Geometry: final body of the model. Coordinates: model frame, mm. A direction names the side the tool comes from. Round coordinates to 2 decimals unless told otherwise and drop trailing zeros. Write each loop counter-clockwise with the first axis right and the second up, starting at its lowest first coordinate (ties: lowest second). Pieces come first, ordered by that corner, then holes. Notation, with made-up numbers: (38.5, 73.5) -> (85.5, 73.5) arc R22 cw to (85.5, 91.5) -> close; hole circle Ø8 at (27, 78). An arc over 180 degrees is marked (long way). One line per item, written item: value. Start each with the question number.
from build123d import *

# Parameters (mm, degrees)
SKETCH1_W           = 50
SKETCH1_H           = 50
BOSS_EXTRUDE1_DEPTH = 2
BOSS_EXTRUDE2_DEPTH = 8
FILLET1_R           = 10
CUT_EXTRUDE1_DEPTH  = 1


with BuildPart() as part:
    # Sketch1 → Boss-Extrude1 (new body)
    with BuildSketch(Plane(origin=(0, 0, 0), x_dir=(1, 0, 0), z_dir=(0, 1, 0))):
        with Locations((-178.886902591, -23.537255169)):
            Rectangle(SKETCH1_W, SKETCH1_H)
    extrude(amount=BOSS_EXTRUDE1_DEPTH)

    # Sketch2 → Boss-Extrude2 (add)
    with BuildSketch(Plane(origin=(0, 2, 0), x_dir=(1, 0, 0), z_dir=(0, 1, 0))):
        with BuildLine():
            Line((-189.683230088, -36.437255169), (-193.090575095, -36.437255169))
            ThreePointArc((-193.090575095, -36.437255169), (-191.386902591, -37.787255169), (-189.683230088, -36.437255169))
        make_face()
        with BuildLine():
            Line((-193.090575095, -35.637255169), (-191.386902591, -35.637255169))
            Line((-191.386902591, -35.637255169), (-189.683230088, -35.637255169))
            ThreePointArc((-189.683230088, -35.637255169), (-191.386902591, -34.287255169), (-193.090575095, -35.637255169))
        make_face()
        with BuildLine():
            Line((-168.090575095, -35.637255169), (-166.386902591, -35.637255169))
            Line((-166.386902591, -35.637255169), (-164.683230088, -35.637255169))
            ThreePointArc((-164.683230088, -35.637255169), (-166.386902591, -34.287255169), (-168.090575095, -35.637255169))
        make_face()
        with BuildLine():
            Line((-164.683230088, -36.437255169), (-168.090575095, -36.437255169))
            ThreePointArc((-168.090575095, -36.437255169), (-166.386902591, -37.787255169), (-164.683230088, -36.437255169))
        make_face()
        with BuildLine():
            Line((-193.346494385, -10.637255169), (-191.386902591, -10.637255169))
            Line((-191.386902591, -10.637255169), (-189.427310797, -10.637255169))
            ThreePointArc((-189.427310797, -10.637255169), (-191.386902591, -9.037255169), (-193.346494385, -10.637255169))
        make_face()
        with BuildLine():
            Line((-189.427310797, -11.437255169), (-193.346494385, -11.437255169))
            ThreePointArc((-193.346494385, -11.437255169), (-191.386902591, -13.037255169), (-189.427310797, -11.437255169))
        make_face()
        with BuildLine():
            Line((-168.346494385, -10.637255169), (-166.386902591, -10.637255169))
            Line((-166.386902591, -10.637255169), (-164.427310797, -10.637255169))
            ThreePointArc((-164.427310797, -10.637255169), (-166.386902591, -9.037255169), (-168.346494385, -10.637255169))
        make_face()
        with BuildLine():
            Line((-164.427310797, -11.437255169), (-168.346494385, -11.437255169))
            ThreePointArc((-168.346494385, -11.437255169), (-166.386902591, -13.037255169), (-164.427310797, -11.437255169))
        make_face()
    extrude(amount=BOSS_EXTRUDE2_DEPTH)

    # Fillet1
    fillet1_edges = [part.edges().sort_by_distance(p)[0] for p in [
        (-203.886902591, 1, -1.462744831),
        (-153.886902591, 1, -1.462744831),
        (-153.886902591, 1, 48.537255169),
        (-203.886902591, 1, 48.537255169),
    ]]
    fillet(fillet1_edges, radius=FILLET1_R)

    # Sketch3 → Cut-Extrude1 (cut)
    with BuildSketch(Plane(origin=(0, 2, 0), x_dir=(1, 0, 0), z_dir=(0, 1, 0))):
        Polygon((-177.886902591, -47.537255169), (-178.886902591, -47.537255169), (-179.886902591, -47.537255169), (-179.886902591, -48.537255169), (-177.886902591, -48.537255169), align=None)
    extrude(amount=-CUT_EXTRUDE1_DEPTH, mode=Mode.SUBTRACT)


solid = part.part
(1) Pin query (flat end, axial travel): pin 1 (3.5 mm diameter, centred on x = -191, y = 5, fed in from +Z); pin 2 (0.8 mm diameter, centred on y = 1.5, z = 48, fed in from -X); pin 3 (4 mm diameter, centred on x = -174.5, y = 4.5, fed in from -Z); pin 4 (1 mm diameter, centred on y = 3.5, z = 34, fed in from +X). Return the tip coordinate at first contact, or that it passes through.
(2) Section query B-B (z = 31.5). Output: boundary loops of the cut face in (x, y), and give its area (3 significant figures).
(3) Section query A-A (y = 8.5). Output: boundary loops of the cut face in (x, z).
(4) Pull-direction query (Z, two-part tool) for faces 1 (the face through (-179, 1, -1.463)), 2 (the face through (-191.354, 5.944, 34.288)), 3 (the face through (-166, 10, 35)), 4 (the face through (-201.035, 1.014, 45.53)); classes: pulls with the +Z half, pulls with the -Z half, needs draft (parallel to the pull), parting line crosses it, or undercut.
(5) Section query C-C (x = -180.5). Output: boundary loops of the cut face in (y, z).
(6) Set-up query: faces 5 (the face through (-191, 6, 13)), 6 (the face through (-179.1, 0.8, 48.537)), 7 (the face through (-191, 6, 36.437)). Return all of +Z, -Z, +X, -X, +Y, -Y with unobstructed straight access to the full face (end or side cutting, diameter ignored); none if empty.
(7) Line query: probe 1 along Z at (x, y) = (-192, 4.75); probe 2 along Y at (x, z) = (-183.5, 16); probe 3 along Z at (x, y) = (-167.5, 6). Output: solid intervals per line, ascending.
Results list:
1. pin 1: stops at z = 37.79
1. pin 2: stops at x = -198.11
1. pin 3: passes through
1. pin 4: stops at x = -165.55
2. outline: (-203.89, 0) -> (-153.89, 0) -> (-153.89, 2) -> (-203.89, 2) -> close
2. area: 100 mm^2
3. outline: (-193.35, 10.64) arc R2 ccw to (-189.43, 10.64) -> close; (-193.35, 11.44) -> (-189.43, 11.44) arc R2 ccw to start; (-193.09, 35.64) arc R1.75 ccw to (-189.68, 35.64) -> close; (-193.09, 36.44) -> (-189.68, 36.44) arc R1.75 ccw to start; (-168.35, 10.64) arc R2 ccw to (-164.43, 10.64) -> close; (-168.35, 11.44) -> (-164.43, 11.44) arc R2 ccw to start; (-168.09, 35.64) arc R1.75 ccw to (-164.68, 35.64) -> close; (-168.09, 36.44) -> (-164.68, 36.44) arc R1.75 ccw to start
4. face 1: pulls with the -Z half
4. face 2: undercut
4. face 3: needs draft
4. face 4: pulls with the +Z half
5. outline: (0, -1.46) -> (2, -1.46) -> (2, 48.54) -> (0, 48.54) -> close
6. face 5: +Y
6. face 6: +Z, +X, -X, +Y, -Y
6. face 7: +X, -X, +Y
7. probe 1: z = 9.13 to 10.64, 11.44 to 12.94, 34.4 to 35.64, 36.44 to 37.68
7. probe 2: y = 0 to 2
7. probe 3: z = 9.38 to 10.64, 11.44 to 12.7, 34.69 to 35.64, 36.44 to 37.39
